Work out the finished part from the listing and answer in its coordinate system (mm). A direction names the side the tool comes from. Coordinates: 2 decimals unless noted, no trailing zeros. Write each loop counter-clockwise with the first axis right and the second up, starting at its lowest first coordinate (ties: lowest second). Pieces come first, ordered by that corner, then holes. Notation, with made-up numbers: (25.25, 70) - (50.25, 70) arc R12 cw to (50.25, 84) - close; hole circle Ø5 at (31, 63). An arc over 180 degrees is marked (long way). One line per item, written item: value.
```python
from build123d import *

# Parameters (mm, degrees)
BOSS_EXTRUDE1_DEPTH = 12.7
SKETCH2_R           = 2.5
CUT_EXTRUDE1_DEPTH  = 16.24
SKETCH3_W           = 7.62
SKETCH3_H           = 3.81
CUT_EXTRUDE2_DEPTH  = 87.4400001


with BuildPart() as part:
    # Sketch1 → Boss-Extrude1 (new body)
    with BuildSketch(Plane.XY):
        with BuildLine():
            Line((-43.22, 0), (43.22, 0))
            Line((43.22, 0), (43.22, -15.24))
            ThreePointArc((43.22, -15.24), (0, -11.337812964), (-43.22, -15.24))
            Line((-43.22, -15.24), (-43.22, 0))
        make_face()
    extrude(amount=BOSS_EXTRUDE1_DEPTH)

    # Sketch2 → Cut-Extrude1 (cut, through all)
    with BuildSketch(Plane(origin=(0, 0, 0), x_dir=(1, 0, 0), z_dir=(0, 1, 0))):
        with Locations((-36.22, -6.35)):
            Circle(SKETCH2_R)
        with Locations((36.22, -6.35)):
            Circle(SKETCH2_R)
    extrude(amount=-CUT_EXTRUDE1_DEPTH, mode=Mode.SUBTRACT)

    # Sketch3 → Cut-Extrude2 (cut, through all)
    with BuildSketch(Plane(origin=(43.22, 0, 0), x_dir=(0, 0, -1), z_dir=(1, 0, 0))):
        with Locations((-6.35, -13.335)):
            Rectangle(SKETCH3_W, SKETCH3_H)
    extrude(amount=-CUT_EXTRUDE2_DEPTH, mode=Mode.SUBTRACT)


solid = part.part
```
Item 1: Which of the six approach directions +Z, -Z, +X, -X, +Y, -Y give full straight-line access (tool end or side, diameter ignored) to faces 5 (the face through (-33.91, -5.63, 7.31)), 6 (the face through (-25, -11.43, 6))?
Evaluation:
face 5: +Y, -Y
face 6: +X, -X, -Y
Item 2: Determine the mould class of faces 1 (the face through (33, -13, 10.16)), 2 (the face through (-43.22, -8, 6)), 3 (the face through (38.53, -5.63, 7.31)), 4 (the face through (0.61, -11.34, 6.26)) for opening direction X: +X half, -X half, draft (parallel to the pull), parting line (faces both ways), or undercut.
Evaluation:
face 1: draft
face 2: -X half
face 3: undercut
face 4: undercut
Item 3: Consider probe 1 along X at (y, z) = (-4.75, 6.35); probe 2 along Z at (x, y) = (36.22, -4.25); probe 3 along X at (y, z) = (-10.75, 8.5). Determine where each line is inside the solid, lowest interval first.
Evaluation:
probe 1: x = -43.22 to -38.72, -33.72 to 33.72, 38.72 to 43.22
probe 2: z = 0 to 3.85, 8.85 to 12.7
probe 3: x = -43.22 to -37.5, -34.94 to 34.94, 37.5 to 43.22
Item 4: Given pin 1 (6 mm diameter, centred on x = 16.5, z = 5, fed in from -Y); pin 2 (2.5 mm diameter, centred on x = -30, z = 4.5, fed in from -Y); pin 3 (6 mm diameter, centred on x = -11.5, z = 3.5, fed in from -Y), each flat-ended and moving along its own axis, determine where each tip first touches the part or whether it passes through.
Evaluation:
pin 1: stops at y = -12.03
pin 2: stops at y = -11.43
pin 3: stops at y = -11.76
Item 5: Section D-D, the plane x = -25.5 is taken. Determine the outline of the cut face in (y, z), then the cut area to 3 significant figures.
Evaluation:
outline: (-12.69, 0) - (0, 0) - (0, 12.7) - (-12.69, 12.7) - (-12.69, 10.16) - (-11.43, 10.16) - (-11.43, 2.54) - (-12.69, 2.54) - close
area: 152 mm2
Item 6: Section B-B, the plane x = -36 is taken. Determine the outline of the cut face in (y, z), then the cut area to 3 significant figures.
Evaluation:
outline: (-14.04, 0) - (0, 0) - (0, 3.86) - (-11.43, 3.86) - (-11.43, 2.54) - (-14.04, 2.54) - close; (-14.04, 10.16) - (-11.43, 10.16) - (-11.43, 8.84) - (0, 8.84) - (0, 12.7) - (-14.04, 12.7) - close
area: 101 mm2
Item 7: Section C-C, the plane y = -6.75 is taken. Determine the outline of the cut face in (x, z).
Evaluation:
outline: (-43.22, 0) - (43.22, 0) - (43.22, 12.7) - (-43.22, 12.7) - close; hole circle Ø5 at (-36.22, 6.35); hole circle Ø5 at (36.22, 6.35)
Item 8: Section A-A, the plane z = 6.35 is taken. Determine the outline of the cut face in (x, y), then the cut area to 3 significant figures.
Evaluation:
outline: (-43.22, -11.43) - (-38.72, -11.43) - (-38.72, 0) - (-43.22, 0) - close; (-33.72, -11.43) - (-6.67, -11.43) arc R241.3 cw to (6.67, -11.43) - (33.72, -11.43) - (33.72, 0) - (-33.72, 0) - close; (38.72, -11.43) - (43.22, -11.43) - (43.22, 0) - (38.72, 0) - close
area: 873 mm2
